The listing builds one solid part. Answer for the finished solid, in the listing's coordinates (mm). Face numbers are marked on the shaded views. A direction names the side the tool comes from. Round coordinates to 2 decimals unless told otherwise and drop trailing zeros. Write each loop counter-clockwise with the first axis right and the second up, starting at its lowest first coordinate (ties: lowest second). Pieces come first, ordered by that corner, then holes. Notation, with made-up numbers: (5, 25.25) - (61, 25.25) arc R26 cw to (61, 53.25) - close; hole circle Ø5 at (61.5, 33). An arc over 180 degrees is marked (long way). Return JSON: item names as keys, results as strings. Group by question number.
(1) Determine the mould class of the marked faces 4, 5 and 6 for opening direction Z: +Z half, -Z half, draft (parallel to the pull), parting line (faces both ways), or undercut.
(2) Each of these flat-tipped pins is pushed along its axis until it touches: pin 1 (8 mm diameter, centred on x = 630.5, y = 421.5, fed in from -Z); pin 2 (2 mm diameter, centred on x = 711, z = 86, fed in from +Y); pin 3 (3 mm diameter, centred on x = -795.5, y = 364.5, fed in from +Z). Where does it stop, or does it pass through?
(3) Which of the six approach directions +Z, -Z, +X, -X, +Y, -Y give full straight-line access (tool end or side, diameter ignored) to the marked faces 1, 2 and 3?
(4) Section B-B, the plane y = -140.5 is taken. Write down the section's boundary in (x, z).
(5) Find the intervals of material crossed by line 1 along Y through (x, z) = (-682, 66.5); line 2 along Y through (x, z) = (112, -143); line 3 along Z through (x, y) = (733, 324), in increasing order. Write a range as [from, to].
(6) Section A-A, the plane x = -351 is taken. Write down the section's boundary in (y, z), then the cut area to 3 significant figures.
(7) Section C-C, the plane y = -698 is taken. Write down the section's boundary in (x, z), then the cut area to 3 significant figures.
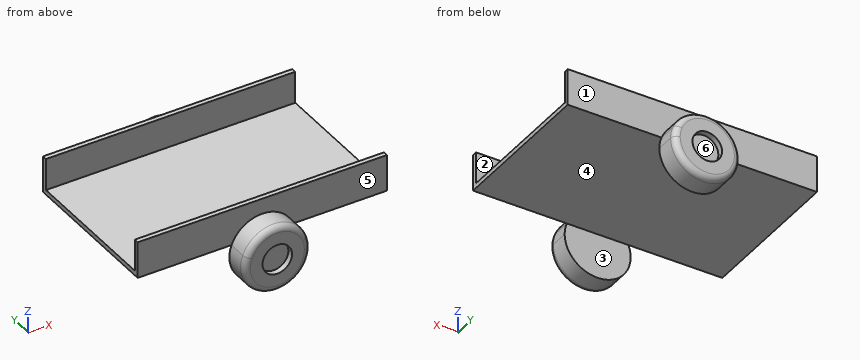
```python
from build123d import *

# Parameters (mm, degrees)
F0_W     = 2110
F0_H     = 1290
F1_DEPTH = 310
F2_T     = -40
F4_DEPTH = 203.2
F5_R     = 50
F6_R     = 125
F7_DEPTH = 50


with BuildPart() as f1:
    # F0 (on Top) → F1 (new body)
    with BuildSketch(Plane.XY):
        Rectangle(F0_W, F0_H)
    extrude(amount=F1_DEPTH)

    # F2
    f2_openings = [f1.faces().sort_by_distance(p)[0] for p in [
        (1055, 0, 155),
        (0, 0, 310),
        (-1055, 0, 155),
    ]]
    offset(amount=F2_T, openings=f2_openings)

    # F3 (on face) → F4 (join)
    with BuildSketch(Plane.XZ.offset(645)):
        with BuildLine():
            Line((-260.891472, 0), (260.891472, 0))
            ThreePointArc((260.891472, 0), (0, 179.4), (-260.891472, 0))
        make_face()
        with BuildLine():
            ThreePointArc((-260.891472, 0), (-50.849203, -374.733905), (279.4, -100))
            ThreePointArc((279.4, -100), (274.733905, -49.150797), (260.891472, 0))
            Line((260.891472, 0), (-260.891472, 0))
        make_face()
    extrude(amount=F4_DEPTH)

    # F5
    f5_edges = [f1.edges().sort_by_distance(p)[0] for p in [
        (-279.4, -848.2, -100),
    ]]
    fillet(f5_edges, radius=F5_R)

    # F6 (on face) → F7 (cut)
    with BuildSketch(Plane.XZ.offset(848.2)):
        with Locations((0, -100)):
            Circle(F6_R)
    extrude(amount=-F7_DEPTH, mode=Mode.SUBTRACT)

    # F8: F1 across plane


with BuildPart() as f1_1:
    add(f1.part)
    add(f1.part.mirror(Plane.XZ))


solid = f1_1.part
```
Working result:
{
 "1": {"face 4": "-Z half", "face 5": "draft", "face 6": "undercut"},
 "2": {"pin 1": "stops at z = 0", "pin 2": "stops at y = 645", "pin 3": "stops at z = 40"},
 "3": {"face 1": "+Z, +Y", "face 2": "+Z, +X, -X", "face 3": "-Z, +X, -X"},
 "4": {"outline": "(-1055, 0) - (1055, 0) - (1055, 40) - (-1055, 40) - close"},
 "5": {"line 1": "y = [-645, -605], [605, 645]", "line 2": "y = [-798.2, -645], [645, 798.2]", "line 3": "z = [0, 40]"},
 "6": {"outline": "(-645, 0) - (645, 0) - (645, 310) - (605, 310) - (605, 40) - (-605, 40) - (-605, 310) - (-645, 310) - close", "area": "73,200 mm^2"},
 "7": {"outline": "(260.89, 0) arc R279.4 ccw (long way) to (279.4, -100) arc R279.4 ccw to start", "area": "245,000 mm^2"}
}
